Read the model definition and answer for the solid it produces. Units are mm, in the model's axes. Face numbers are marked on the shaded views. A direction names the side the tool comes from. Coordinates: 2 decimals unless noted, no trailing zeros. Loops run counter-clockwise (first coordinate to the right, second up) from the corner with the lowest first, then second, coordinate; pieces in that order, holes last.
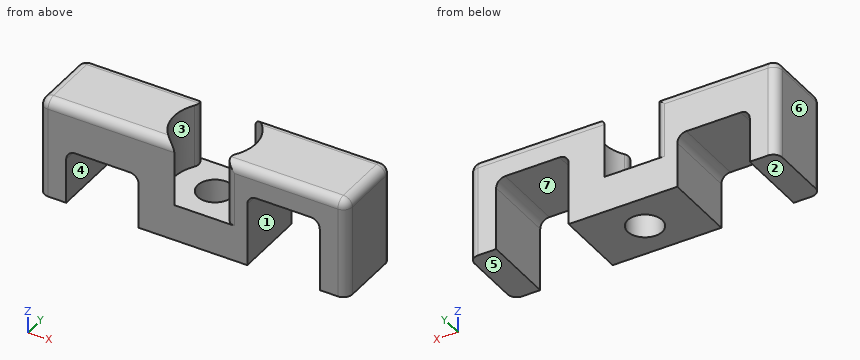
Autodesk Inventor part; units mm, degrees
ref_plane "YZ Plane" through (0, 0, 0) normal (1, 0, 0) x (0, 1, 0)
ref_plane "XZ Plane" through (0, 0, 0) normal (0, 1, 0) x (-1, 0, 0)
ref_plane "XY Plane" through (0, 0, 0) normal (0, 0, 1) x (1, 0, 0)
sketch "Sketch1" plane through (0, 0, 0) normal (0, 0, 1) x (1, 0, 0)
  line L0 (0, 4) -> (16, 4)
  line L1 (17, 3) -> (17, -3)
  line L2 (16, -4) -> (0, -4)
  arc A0 (17, 3) -> (16, 4) centre (16, 3) ccw
  arc A1 (16, -4) -> (17, -3) centre (16, -3) ccw
  line L3 (0, 4) -> (-16, 4)
  line L4 (-17, 3) -> (-17, -3)
  line L5 (-16, -4) -> (0, -4)
  arc A2 (-16, 4) -> (-17, 3) centre (-16, 3) ccw
  arc A3 (-17, -3) -> (-16, -4) centre (-16, -3) ccw
  line L6 (0, 4) -> (0, -4)
  point P0 (0, 0)
  point P1 (0, 0)
  dimension "d1" = 17
  dimension "d2" = 1
  dimension "d17" = 17
  dimension "d18" = 4
  dimension "d19" = 4
  dimension "d20" = 1
  dimension "d21" = 8
  dimension "d22" = 4
extrude "Extrusion1" add sketch "Sketch1" along normal blind 11
sketch "Sketch5" plane through (-16, -4, 0) normal (0, -1, 0) x (1, 0, 0)
  line L0 (0, 0) -> (32, 0)
  line L1 (22, 0) -> (30, 0)
  line L2 (30, 0) -> (30, 7)
  line L3 (29, 8) -> (23, 8)
  line L4 (22, 7) -> (22, 0)
  line L5 (33, 0) -> (33, 11)
  arc A0 (23, 8) -> (22, 7) centre (23, 7) ccw
  arc A1 (30, 7) -> (29, 8) centre (29, 7) ccw
  line L6 (3, 6) -> (9, 6)
  line L7 (10, 5) -> (10, 0)
  line L8 (10, 0) -> (2, 0)
  line L9 (2, 0) -> (2, 5)
  line L10 (-1, 0) -> (-1, 11)
  line L11 (32, 0) -> (0, 0)
  arc A2 (3, 6) -> (2, 5) centre (3, 5) ccw
  arc A3 (10, 5) -> (9, 6) centre (9, 5) ccw
  point P0 (16, 0)
  point P1 (10, 6)
  dimension "d28" = 3
  dimension "d29" = 8
  dimension "d30" = 8
  dimension "d31" = 1
  dimension "d34" = 3
  dimension "d35" = 8
  dimension "d36" = 6
  dimension "d37" = 1
extrude "Extrusion5" cut sketch "Sketch5" against normal through all
sketch "Sketch3" plane through (-16, -3, 11) normal (0, 0, 1) x (1, 0, 0)
  circle A0 centre (16, 3) radius 4.5
  dimension "d38" = 9
extrude "Extrusion3" cut sketch "Sketch3" against normal blind 7
sketch "Sketch4" plane through (-16, -3, 4) normal (0, 0, 1) x (1, 0, 0)
  circle A0 centre (16, 3) radius 1.905
  dimension "d13" = 3.81
extrude "Extrusion4" cut sketch "Sketch4" against normal through all
fillet "Fillet2" radius 1 10 edges at (9.0308, -4, 11) (-16.7071, -3.7071, 11) (-17, 0, 11) (-16.7071, 3.7071, 11) (-9.0308, 4, 11) (16.7071, -3.7071, 11) (17, 0, 11) (16.7071, 3.7071, 11) (2.0616, -4, 7.5) (-2.0616, 4, 7.5)
properties part number "WireClampDual"
Q1. Determine the mould class of the marked faces 4, 5, 6 and 7 for opening direction X: +X half, -X half, draft (parallel to the pull), parting line (faces both ways), or undercut.
Findings below:
face 4: undercut
face 5: draft
face 6: -X half
face 7: undercut
Q2. Straight lines are drawn through the part: probe 1 along X at (y, z) = (2.75, 2); probe 2 along X at (y, z) = (1.25, 0.5); probe 3 along Y at (x, z) = (0, 1.9) (3 decimals). For each, find the intervals that lie inside material, in ascending order.
Findings below:
probe 1: x = -17 to -14, -6 to 6, 14 to 17
probe 2: x = -17 to -14, -6 to -1.44, 1.44 to 6, 14 to 17
probe 3: y = -4 to -1.905, 1.905 to 4
Q3. A cutting plane is placed at D-D (x = 9). Give the vertices of the cut face in (y, z).
Findings below:
outline: (-4, 8) - (4, 8) - (4, 10) arc R1 ccw to (3, 11) - (-3, 11) arc R1 ccw to (-4, 10) - close
Q4. A cutting plane is placed at C-C (y = 0). Give the vertices of the cut face in (x, z) (3 decimals).
Findings below:
outline: (-17, 0) - (-14, 0) - (-14, 5) arc R1 cw to (-13, 6) - (-7, 6) arc R1 cw to (-6, 5) - (-6, 0) - (-1.905, 0) - (-1.905, 4) - (-4.5, 4) - (-4.5, 11) - (-16, 11) arc R1 ccw to (-17, 10) - close; (1.905, 0) - (6, 0) - (6, 7) arc R1 cw to (7, 8) - (13, 8) arc R1 cw to (14, 7) - (14, 0) - (17, 0) - (17, 10) arc R1 ccw to (16, 11) - (4.5, 11) - (4.5, 4) - (1.905, 4) - close
Q5. Which of the six approach directions +Z, -Z, +X, -X, +Y, -Y give full straight-line access (tool end or side, diameter ignored) to the marked faces 1, 2 and 3?
Findings below:
face 1: -Z, +Y, -Y
face 2: -Z, +X, -X, +Y, -Y
face 3: +Z
Q6. A cutting plane is placed at B-B (z = 1.75). Give the vertices of the cut face in (x, y) (3 decimals).
Findings below:
outline: (-17, -3) arc R1 ccw to (-16, -4) - (-14, -4) - (-14, 4) - (-16, 4) arc R1 ccw to (-17, 3) - close; (-6, -4) - (6, -4) - (6, 4) - (-6, 4) - close; (14, -4) - (16, -4) arc R1 ccw to (17, -3) - (17, 3) arc R1 ccw to (16, 4) - (14, 4) - close; hole circle Ø3.81 at (0, 0)
Q7. A cutting plane is placed at A-A (x = 0). Give the vertices of the cut face in (y, z) (3 decimals), then the cut area to 3 significant figures.
Findings below:
outline: (-4, 0) - (-1.905, 0) - (-1.905, 4) - (-4, 4) - close; (1.905, 0) - (4, 0) - (4, 4) - (1.905, 4) - close
area: 16.8 mm2
Q8. Flat-ended cylindrical pins translate along their axes: pin 1 Ø1 at (x, y) = (3, 0) entering from +Z; pin 2 Ø1.8 at (x, y) = (-11.5, 1) entering from -Z. Find the tip coordinate at first contact, or state that the pin passes through.
Findings below:
pin 1: stops at z = 4
pin 2: stops at z = 6
